Input: part model. Units: mm. Frame: model coordinates. A direction names the side the tool comes from. Round coordinates to 2 decimals unless told otherwise and drop trailing zeros. Order: outer loops, then holes, each group sorted by start corner. A loop starts at its lowest first (then second) coordinate and runs counter-clockwise, first axis right, second up. Notation, with made-up numbers: (38, 76.5) -> (44, 76.5) arc R13 cw to (44, 88.5) -> close; hole circle Ø6 at (74, 35). An arc over 180 degrees is marked (long way). Answer as CSV lines item,"result". Start each with the question number.
1) Mould query, pull axis Z, two halves, no side actions, for faces 4 (the face through (-0.4, 25, 0.9)), 5 (the face through (6, 0, 25.4)), 6 (the face through (-0.32, -21.55, 0.43)), 7 (the face through (-0.32, 24.43, -24.8)). Classes: +Z half, -Z half, draft (parallel to the pull), parting line (faces both ways), or undercut.
2) Section query D-D, the plane y = 1. Output: boundary loops of the cut face in (x, z) (3 decimals), and give its area (3 significant figures).
3) First-contact query: P1, Ø24.5, axis at y = 1.5, z = 4.5, coming from the +X side; P2, Ø0.5, axis at x = -0.5, y = 8, coming from the +Z side; P3, Ø0.7, axis at x = -0.5, y = -6.5, coming from the +Z side. Flat tips, straight axial feed; report the tip coordinate or a pass-through.
4) Section query C-C, the plane x = 5. Output: boundary loops of the cut face in (y, z) (3 decimals), and give its area (3 significant figures).
5) Section query A-A, the plane y = 8. Output: boundary loops of the cut face in (x, z) (3 decimals).
6) Line query: L1, parallel to X at y = 22, z = 20 (3 decimals); L2, parallel to Z at x = 6.5, y = 17 (3 decimals). Output: solid intervals per line, ascending.
7) Section query B-B, the plane z = 0.4. Output: boundary loops of the cut face in (x, y) (3 decimals), and give its area (3 significant figures).
8) Access query for faces 1 (the face through (-0.32, 10.05, 0.37)), 2 (the face through (0, 0, -6)), 3 (the face through (10.764, -24.43, 25.078)). Directions: +Z, -Z, +X, -X, +Y, -Y. A direction counts if a zero-diameter tool reaches every point of the face in a straight line with its end or side. Return the directions, or none.
```python
from build123d import *

# Parameters (mm, degrees)
SKETCH1_W                    = 50.8
SKETCH1_H                    = 50
BASE_FLANGE1_DEPTH           = 0.635
SKETCH9_W                    = 12
SKETCH9_H                    = 24.6
CUT_EXTRUDE1_DEPTH           = 36.644960724
CUT_EXTRUDE2_DEPTH           = 36.644960724
EDGE_FLANGE1_STRIP_W         = 4.54
EDGE_FLANGE1_STRIP_H         = 0.635
EDGE_FLANGE1_STRIP_CUT_DEPTH = 50
EDGE_FLANGE1_DEPTH           = 50
SKETCH14_R                   = 2.65
CUT_EXTRUDE3_DEPTH           = 58.189950603
FILLET1_R                    = 2


# Sheet-metal steps are written as plain solids
with BuildPart() as part:
    # Sketch1 → Base-Flange1 (new body)
    with BuildSketch(Plane(origin=(0, 0, 0), x_dir=(0, 0, -1), z_dir=(1, 0, 0))):
        Rectangle(SKETCH1_W, SKETCH1_H)
    extrude(amount=-BASE_FLANGE1_DEPTH)

    # Sketch9 → Cut-Extrude1 (cut, through all)
    with BuildSketch(Plane(origin=(0, 0, 0), x_dir=(0, 0, -1), z_dir=(1, 0, 0))):
        with Locations((-0.3, -5.75)):
            Rectangle(SKETCH9_W, SKETCH9_H)
    extrude(amount=-CUT_EXTRUDE1_DEPTH, mode=Mode.SUBTRACT)

    # Sketch10 → Cut-Extrude2 (cut, through all)
    with BuildSketch(Plane.ZY.offset(0.635)):
        with BuildLine():
            Line((-0.75, -20.4), (-0.75, -18.4))
            ThreePointArc((-0.75, -18.4), (0.4, -17.25), (1.55, -18.4))
            Line((1.55, -18.4), (1.55, -20.4))
            ThreePointArc((1.55, -20.4), (0.4, -21.55), (-0.75, -20.4))
        make_face()
        with BuildLine():
            Line((-0.75, 6.9), (-0.75, 8.9))
            ThreePointArc((-0.75, 8.9), (0.4, 10.05), (1.55, 8.9))
            Line((1.55, 8.9), (1.55, 6.9))
            ThreePointArc((1.55, 6.9), (0.4, 5.75), (-0.75, 6.9))
        make_face()
    extrude(amount=-CUT_EXTRUDE2_DEPTH, mode=Mode.SUBTRACT)

    # Edge-Flange1 strip (across the edge) → Edge-Flange1 strip cut (cut)
    with BuildSketch(Plane(origin=(0, 25, 25.4), x_dir=(0, 0, -1), z_dir=(0, -1, 0))):
        with Locations((-0.635, -0.3175)):
            Rectangle(EDGE_FLANGE1_STRIP_W, EDGE_FLANGE1_STRIP_H)
    extrude(amount=EDGE_FLANGE1_STRIP_CUT_DEPTH, mode=Mode.SUBTRACT)

    # Edge-Flange1 section (across the edge) → Edge-Flange1 (add)
    with BuildSketch(Plane(origin=(0, 25, 25.4), x_dir=(0, 0, -1), z_dir=(0, -1, 0))):
        with BuildLine():
            Line((0, 1), (0, 11.365))
            Line((0, 11.365), (0.635, 11.365))
            Line((0.635, 11.365), (0.635, 1))
            ThreePointArc((0.635, 1), (0.927893219, 0.292893219), (1.635, 0))
            Line((1.635, 0), (1.635, -0.635))
            ThreePointArc((1.635, -0.635), (0.478880413, -0.156119587), (0, 1))
        make_face()
    extrude(amount=EDGE_FLANGE1_DEPTH)

    # Sketch14 → Cut-Extrude3 (cut, through all)
    with BuildSketch(Plane(origin=(0, 0, 24.765), x_dir=(-1, 0, 0), z_dir=(0, 0, -1))):
        with Locations((-6.1825, -20)):
            Circle(SKETCH14_R)
        with Locations((-6.1825, 20)):
            Circle(SKETCH14_R)
    extrude(amount=-CUT_EXTRUDE3_DEPTH, mode=Mode.SUBTRACT)

    # Fillet1
    fillet1_edges = [part.edges().sort_by_distance(p)[0] for p in [
        (11.365, 25, 25.0825),
        (11.365, -25, 25.0825),
        (-0.3175, -25, -25.4),
        (-0.3175, 25, -25.4),
    ]]
    fillet(fillet1_edges, radius=FILLET1_R)


solid = part.part
```
Findings:
1,face 4,"draft"
1,face 5,"+Z half"
1,face 6,"undercut"
1,face 7,"-Z half"
2,outline,"(-0.635, -25.4) -> (0, -25.4) -> (0, -5.7) -> (-0.635, -5.7) -> close; (-0.635, 6.3) -> (0, 6.3) -> (0, 23.765) arc R1 cw to (1, 24.765) -> (11.365, 24.765) -> (11.365, 25.4) -> (1, 25.4) arc R1.635 ccw to (-0.635, 23.765) -> close"
2,area,"31.5 mm^2"
3,P1,"stops at x = 0"
3,P2,"stops at z = 24.82"
3,P3,"stops at z = 24.93"
4,outline,"(-25, 24.765) -> (-22.372, 24.765) -> (-22.372, 25.4) -> (-25, 25.4) -> close; (-17.628, 24.765) -> (17.628, 24.765) -> (17.628, 25.4) -> (-17.628, 25.4) -> close; (22.372, 24.765) -> (25, 24.765) -> (25, 25.4) -> (22.372, 25.4) -> close"
4,area,"25.7 mm^2"
5,outline,"(-0.635, -25.4) -> (0, -25.4) -> (0, -0.75) -> (-0.635, -0.75) -> close; (-0.635, 1.55) -> (0, 1.55) -> (0, 23.765) arc R1 cw to (1, 24.765) -> (11.365, 24.765) -> (11.365, 25.4) -> (1, 25.4) arc R1.635 ccw to (-0.635, 23.765) -> close"
6,L1,"x = -0.635 to 0"
6,L2,"z = 24.765 to 25.4"
7,outline,"(-0.635, -25) -> (0, -25) -> (0, -21.55) -> (-0.635, -21.55) -> close; (-0.635, 10.05) -> (0, 10.05) -> (0, 25) -> (-0.635, 25) -> close"
7,area,"11.7 mm^2"
8,face 1,"+X, -X"
8,face 2,"-Z, +X, +Y, -Y"
8,face 3,"+Z, -Z, +X, -Y"
